Autodesk Inventor part; units mm, degrees
ref_plane "YZ Plane" through (0, 0, 0) normal (1, 0, 0) x (0, 1, 0)
ref_plane "XZ Plane" through (0, 0, 0) normal (0, 1, 0) x (-1, 0, 0)
ref_plane "XY Plane" through (0, 0, 0) normal (0, 0, 1) x (1, 0, 0)
sketch "Sketch1" plane through (0, 0, 0) normal (0, 0, 1) x (1, 0, 0)
  circle A0 centre (-20.1638, -35.1051) radius 1.25
  circle A1 centre (19.9556, 35.1051) radius 1.25
  circle A2 centre (20.3721, -35.1051) radius 1.25
  circle A3 centre (-19.7473, 35.1051) radius 1.25
  arc A4 (-17.1638, -35.1051) -> (-21.6638, -32.507) centre (-20.1638, -35.1051) ccw
  arc A5 (-23.0299, -32.141) -> (-21.6638, -32.507) centre (-22.1638, -31.641) ccw
  line L0 (-23.0299, -32.141) -> (-41.5865, 0)
  line L1 (-41.5865, 0) -> (-22.9176, 32.3355)
  arc A6 (-21.4755, 32.6529) -> (-22.9176, 32.3355) centre (-22.0516, 31.8355) ccw
  arc A7 (-21.4755, 32.6529) -> (-16.7473, 35.1051) centre (-19.7473, 35.1051) ccw
  arc A8 (-15.7473, 36.1051) -> (-16.7473, 35.1051) centre (-15.7473, 35.1051) ccw
  line L2 (-15.7473, 36.1051) -> (15.9556, 36.1051)
  arc A9 (16.9556, 35.1051) -> (15.9556, 36.1051) centre (15.9556, 35.1051) ccw
  arc A10 (16.9556, 35.1051) -> (21.4556, 32.507) centre (19.9556, 35.1051) ccw
  arc A11 (22.8216, 32.141) -> (21.4556, 32.507) centre (21.9556, 31.641) ccw
  line L3 (22.8216, 32.141) -> (41.5865, -0.3607)
  line L4 (41.5865, -0.3607) -> (23.2381, -32.141)
  arc A12 (21.8721, -32.507) -> (23.2381, -32.141) centre (22.3721, -31.641) ccw
  arc A13 (21.8721, -32.507) -> (17.3721, -35.1051) centre (20.3721, -35.1051) ccw
  arc A14 (16.3721, -36.1051) -> (17.3721, -35.1051) centre (16.3721, -35.1051) ccw
  line L5 (16.3721, -36.1051) -> (-16.1638, -36.1051)
  arc A15 (-17.1638, -35.1051) -> (-16.1638, -36.1051) centre (-16.1638, -35.1051) ccw
  line L6 (-43.3185, -1) -> (-22.4732, -37.1051)
  arc A16 (-22.4732, -37.1051) -> (-20.7412, -38.1051) centre (-20.7412, -36.1051) ccw
  line L7 (-20.7412, -38.1051) -> (20.9494, -38.1051)
  arc A17 (20.9494, -38.1051) -> (22.6815, -37.1051) centre (20.9494, -36.1051) ccw
  line L8 (22.6815, -37.1051) -> (43.3185, -1.3607)
  arc A18 (43.3185, -1.3607) -> (43.3185, 0.6393) centre (41.5865, -0.3607) ccw
  line L9 (43.3185, 0.6393) -> (22.265, 37.1051)
  arc A19 (22.265, 37.1051) -> (20.5329, 38.1051) centre (20.5329, 36.1051) ccw
  line L10 (20.5329, 38.1051) -> (-20.7412, 38.1051)
  arc A20 (-20.7412, 38.1051) -> (-22.4732, 37.1051) centre (-20.7412, 36.1051) ccw
  line L11 (-22.4732, 37.1051) -> (-43.3185, 1)
  arc A21 (-43.3185, 1) -> (-43.3185, -1) centre (-41.5865, 0) ccw
  point P0 (0, 0)
extrude "Extrusion1" add sketch "Sketch1" along normal blind 10
sketch "Sketch2" plane through (0, 0, 10) normal (0, 0, 1) x (1, 0, 0)
  arc A0 (19.392, 12.5813) -> (25.0985, 14.4351) centre (22.2452, 13.5082) ccw
  arc A1 (19.392, 12.5813) -> (10.8356, 23.4883) centre (0.2256, 6.3551) ccw
  arc A2 (13.9946, 28.5893) -> (10.8356, 23.4883) centre (12.4151, 26.0388) ccw
  arc A3 (25.0985, 14.4351) -> (13.9946, 28.5893) centre (0.2256, 6.3551) ccw
  arc A4 (-19.0054, -13.2092) -> (-24.656, -15.2268) centre (-21.8307, -14.218) ccw
  arc A5 (-19.0054, -13.2092) -> (-10.7215, -23.5712) centre (0.1909, -6.3551) ccw
  arc A6 (-13.9337, -28.639) -> (-10.7215, -23.5712) centre (-12.3276, -26.1051) ccw
  arc A7 (-24.656, -15.2268) -> (-13.9337, -28.639) centre (0.1909, -6.3551) ccw
  arc A8 (10.216, 9.6769) -> (15.4555, 12.6005) centre (12.8358, 11.1387) ccw
  arc A9 (10.216, 9.6769) -> (5.8047, 15.0962) centre (-7.382, -0.1428) ccw
  arc A10 (9.7308, 19.6334) -> (5.8047, 15.0962) centre (7.7677, 17.3648) ccw
  arc A11 (15.4555, 12.6005) -> (9.7308, 19.6334) centre (-7.382, -0.1428) ccw
  arc A12 (-5.3056, 15.1266) -> (-9.2069, 19.6851) centre (-7.2562, 17.4058) ccw
  arc A13 (-5.3056, 15.1266) -> (-9.7465, 9.7314) centre (7.7976, -0.1843) ccw
  arc A14 (-14.9699, 12.6837) -> (-9.7465, 9.7314) centre (-12.3582, 11.2076) ccw
  arc A15 (-9.2069, 19.6851) -> (-14.9699, 12.6837) centre (7.7976, -0.1843) ccw
  arc A16 (-9.7465, -9.7314) -> (-14.9699, -12.6837) centre (-12.3582, -11.2076) ccw
  arc A17 (-9.7465, -9.7314) -> (-5.3056, -15.1266) centre (7.7976, 0.1843) ccw
  arc A18 (-9.2069, -19.6851) -> (-5.3056, -15.1266) centre (-7.2562, -17.4058) ccw
  arc A19 (-14.9699, -12.6837) -> (-9.2069, -19.6851) centre (7.7976, 0.1843) ccw
  arc A20 (5.6394, -15.1565) -> (9.5156, -19.7363) centre (7.5775, -17.4464) ccw
  arc A21 (5.6394, -15.1565) -> (10.1097, -9.7857) centre (-7.3799, 0.2258) ccw
  arc A22 (15.3169, -12.7664) -> (10.1097, -9.7857) centre (12.7133, -11.2761) ccw
  arc A23 (9.5156, -19.7363) -> (15.3169, -12.7664) centre (-7.3799, 0.2258) ccw
  arc A24 (11.009, -23.6306) -> (14.1935, -28.7158) centre (12.6012, -26.1732) ccw
  arc A25 (11.009, -23.6306) -> (19.3494, -13.314) centre (0.1909, -6.3551) ccw
  arc A26 (24.9889, -15.3625) -> (19.3494, -13.314) centre (22.1691, -14.3383) ccw
  arc A27 (14.1935, -28.7158) -> (24.9889, -15.3625) centre (0.1909, -6.3551) ccw
  arc A28 (-10.2906, 23.546) -> (-13.4216, 28.6643) centre (-11.8561, 26.1051) ccw
  arc A29 (-10.2906, 23.546) -> (-18.9065, 12.686) centre (0.2256, 6.3551) ccw
  arc A30 (-24.6027, 14.5709) -> (-18.9065, 12.686) centre (-21.7546, 13.6284) ccw
  arc A31 (-13.4216, 28.6643) -> (-24.6027, 14.5709) centre (0.2256, 6.3551) ccw
  circle A32 centre (-19.7473, 35.1051) radius 1.25 construction
  circle A33 centre (20.3721, -35.1051) radius 1.25 construction
  circle A34 centre (19.9556, 35.1051) radius 1.25 construction
  circle A35 centre (-20.1638, -35.1051) radius 1.25 construction
  line L0 (-43.1103, 0.6393) -> (-22.0567, 37.1051) construction
  arc A36 (-43.1103, 0.6393) -> (-43.1103, -1.3607) centre (-41.3782, -0.3607) ccw construction
  line L1 (-22.4732, -37.1051) -> (-43.1103, -1.3607) construction
  arc A37 (-22.4732, -37.1051) -> (-20.7412, -38.1051) centre (-20.7412, -36.1051) ccw construction
  line L2 (20.9494, -38.1051) -> (-20.7412, -38.1051) construction
  arc A38 (20.9494, -38.1051) -> (22.6815, -37.1051) centre (20.9494, -36.1051) ccw construction
  line L3 (43.5268, -1) -> (22.6815, -37.1051) construction
  arc A39 (43.5268, -1) -> (43.5268, 1) centre (41.7947, 0) ccw construction
  line L4 (22.6815, 37.1051) -> (43.5268, 1) construction
  arc A40 (22.6815, 37.1051) -> (20.9494, 38.1051) centre (20.9494, 36.1051) ccw construction
  line L5 (-20.3247, 38.1051) -> (20.9494, 38.1051) construction
  arc A41 (-20.3247, 38.1051) -> (-22.0567, 37.1051) centre (-20.3247, 36.1051) ccw construction
  arc A42 (-22.4732, -37.1051) -> (-20.7412, -38.1051) centre (-20.7412, -36.1051) ccw
  line L6 (-20.7412, -38.1051) -> (20.9494, -38.1051)
  arc A43 (20.9494, -38.1051) -> (22.6815, -37.1051) centre (20.9494, -36.1051) ccw
  line L7 (22.6815, -37.1051) -> (43.3185, -1.3607)
  arc A44 (43.3185, -1.3607) -> (43.3185, 0.6393) centre (41.5865, -0.3607) ccw
  line L8 (43.3185, 0.6393) -> (22.265, 37.1051)
  arc A45 (22.265, 37.1051) -> (20.5329, 38.1051) centre (20.5329, 36.1051) ccw
  line L9 (20.5329, 38.1051) -> (-20.7412, 38.1051)
  arc A46 (-20.7412, 38.1051) -> (-22.4732, 37.1051) centre (-20.7412, 36.1051) ccw
  line L10 (-22.4732, 37.1051) -> (-43.3185, 1)
  arc A47 (-43.3185, 1) -> (-43.3185, -1) centre (-41.5865, 0) ccw
  line L11 (-43.3185, -1) -> (-22.4732, -37.1051)
  line L12 (16.3721, -36.1051) -> (-16.1638, -36.1051)
  arc A48 (-17.1638, -35.1051) -> (-16.1638, -36.1051) centre (-16.1638, -35.1051) ccw
  arc A49 (-17.1638, -35.1051) -> (-21.6638, -32.507) centre (-20.1638, -35.1051) ccw
  arc A50 (-23.0299, -32.141) -> (-21.6638, -32.507) centre (-22.1638, -31.641) ccw
  line L13 (-23.0299, -32.141) -> (-41.5865, 0)
  line L14 (-41.5865, 0) -> (-22.9176, 32.3355)
  arc A51 (-21.4755, 32.6529) -> (-22.9176, 32.3355) centre (-22.0516, 31.8355) ccw
  arc A52 (-21.4755, 32.6529) -> (-16.7473, 35.1051) centre (-19.7473, 35.1051) ccw
  arc A53 (-15.7473, 36.1051) -> (-16.7473, 35.1051) centre (-15.7473, 35.1051) ccw
  line L15 (-15.7473, 36.1051) -> (15.9556, 36.1051)
  arc A54 (16.9556, 35.1051) -> (15.9556, 36.1051) centre (15.9556, 35.1051) ccw
  arc A55 (16.9556, 35.1051) -> (21.4556, 32.507) centre (19.9556, 35.1051) ccw
  arc A56 (22.8216, 32.141) -> (21.4556, 32.507) centre (21.9556, 31.641) ccw
  line L16 (22.8216, 32.141) -> (41.5865, -0.3607)
  line L17 (41.5865, -0.3607) -> (23.2381, -32.141)
  arc A57 (21.8721, -32.507) -> (23.2381, -32.141) centre (22.3721, -31.641) ccw
  arc A58 (21.8721, -32.507) -> (17.3721, -35.1051) centre (20.3721, -35.1051) ccw
  arc A59 (16.3721, -36.1051) -> (17.3721, -35.1051) centre (16.3721, -35.1051) ccw
  circle A60 centre (-19.7473, 35.1051) radius 1.25
  circle A61 centre (20.3721, -35.1051) radius 1.25
  circle A62 centre (19.9556, 35.1051) radius 1.25
  circle A63 centre (-20.1638, -35.1051) radius 1.25
  point P0 (0, 0)
  dimension "d4" = 2.5
extrude "Extrusion2" add sketch "Sketch2" along normal blind 4 contours L11 A47 L10 A46 L9 A45 L8 A44 L7 A43 L6 A42 | L12 A48 A49 A50 L13 L14 A51 A52 A53 L15 A54 A55 A56 L16 L17 A57 A58 A59
sketch "Sketch3" plane through (0, 0, 14) normal (0, 0, 1) x (1, 0, 0)
  circle A0 centre (-19.7473, 35.1051) radius 1.25 construction
  circle A1 centre (19.9556, 35.1051) radius 1.25 construction
  circle A2 centre (-20.1638, -35.1051) radius 1.25 construction
  circle A3 centre (20.3721, -35.1051) radius 1.25 construction
  circle A4 centre (-19.7473, 35.1051) radius 1.6
  circle A5 centre (19.9556, 35.1051) radius 1.6
  circle A6 centre (-20.1638, -35.1051) radius 1.6
  circle A7 centre (20.3721, -35.1051) radius 1.6
  point P0 (0, 0)
  dimension "d5" = 3.2
extrude "Extrusion3" cut sketch "Sketch3" against normal through all
properties part number "ArmPowerBoardBack"
Could you check a few things on this model? Use its own coordinates, in mm. A direction names the side the tool comes from. Coordinates: 2 decimals unless noted, no trailing zeros. Write each loop counter-clockwise with the first axis right and the second up, starting at its lowest first coordinate (ties: lowest second). Pieces come first, ordered by that corner, then holes. Notation, with made-up numbers: (65, 30) - (88, 30) arc R24 cw to (88, 64) - close; hole circle Ø2 at (10, 69). An arc over 180 degrees is marked (long way). Put each result on its own line as item: value. Start each with the question number.
Q1. Please list where these lines run through material, in increasing order: L1, parallel to Y at x = -20, z = 4.75; L2, parallel to X at y = -24.5, z = 12; L3, parallel to Y at x = 15.5, z = 9.
Q2. Thinking about a two-plate mould opening in Y: for faces 1 (the cylindrical face through (-13.777, 8.564, 11.972)), 2 (the flat face through (-33.04, -18.8, 6.9)), 3 (the cylindrical face through (-43.586, -0.015, 6.902)), which applies, pulls with the +Y half, pulls with the -Y half, needs draft (parallel to the pull), parting line crosses it, or undercut?
Q3. Which directions (+Z, -Z, +X, -X, +Y, -Y) give clear straight access to the entire face, cutting with the end or side of a thin tool? Please do faces 4 (the cylindrical face through (16.02, 18.87, 11.97)), 5 (the flat face through (32.07, 16.12, 4.93)), 6 (the flat face through (-1, 1, 14)).
Q4. I want a section at A-A on y = -22. Write out the boundary of the cut face in (x, z), plus the area to 3 significant figures.
Q5. I'm going to push flat-ended pins straight in: P1, Ø5, axis at x = 19.96, y = 35.11, coming from the +Z side; P2, Ø6, axis at x = -26.5, y = -13.5, coming from the -Z side; P3, Ø3, axis at x = 32.5, z = 12, coming from the -Y side; P4, Ø1.5, axis at y = 20.5, z = 5.5, coming from the -X side. Where does each tip first touch, or does it pass through?
Q6. I want a section at B-B on x = -6.5. Write out the boundary of the cut face in (y, z).
Q7. I want a section at C-C on z = 12.25. Count the separate pieces of the cut face and the enclosed holes in it, plus the area to 3 significant figures.
Checks:
1. L1: -38.11 to -36.7, -33.51 to -32.11, 32.12 to 33.53, 36.69 to 38.11
1. L2: -29.75 to -18.96, -9.79 to 10.11, 19.34 to 29.96
1. L3: -38.11 to -36.11, 36.11 to 38.11
2. face 1: undercut
2. face 2: pulls with the -Y half
2. face 3: parting line crosses it
3. face 4: +Z, -Z
3. face 5: -Z
3. face 6: +Z, +X, -X, +Y, -Y
4. outline: (-31.19, 0) - (-28.88, 0) - (-28.88, 10) - (-21.05, 10) - (-21.05, 14) - (-31.19, 14) - close; (-12.87, 10) - (13.26, 10) - (13.26, 14) - (-12.87, 14) - close; (21.43, 10) - (29.09, 10) - (29.09, 0) - (31.4, 0) - (31.4, 14) - (21.43, 14) - close
4. area: 231 mm²
5. P1: z = 14
5. P2: z = 10
5. P3: y = -22.7
5. P4: x = -32.49
6. outline: (-38.11, 0) - (-36.11, 0) - (-36.11, 10) - (-20.31, 10) - (-20.31, 14) - (-38.11, 14) - close; (-14.02, 10) - (14.02, 10) - (14.02, 14) - (-14.02, 14) - close; (20.31, 10) - (36.11, 10) - (36.11, 0) - (38.11, 0) - (38.11, 14) - (20.31, 14) - close
7. separate pieces: 1
7. enclosed holes: 12
7. area: 4,180 mm²
